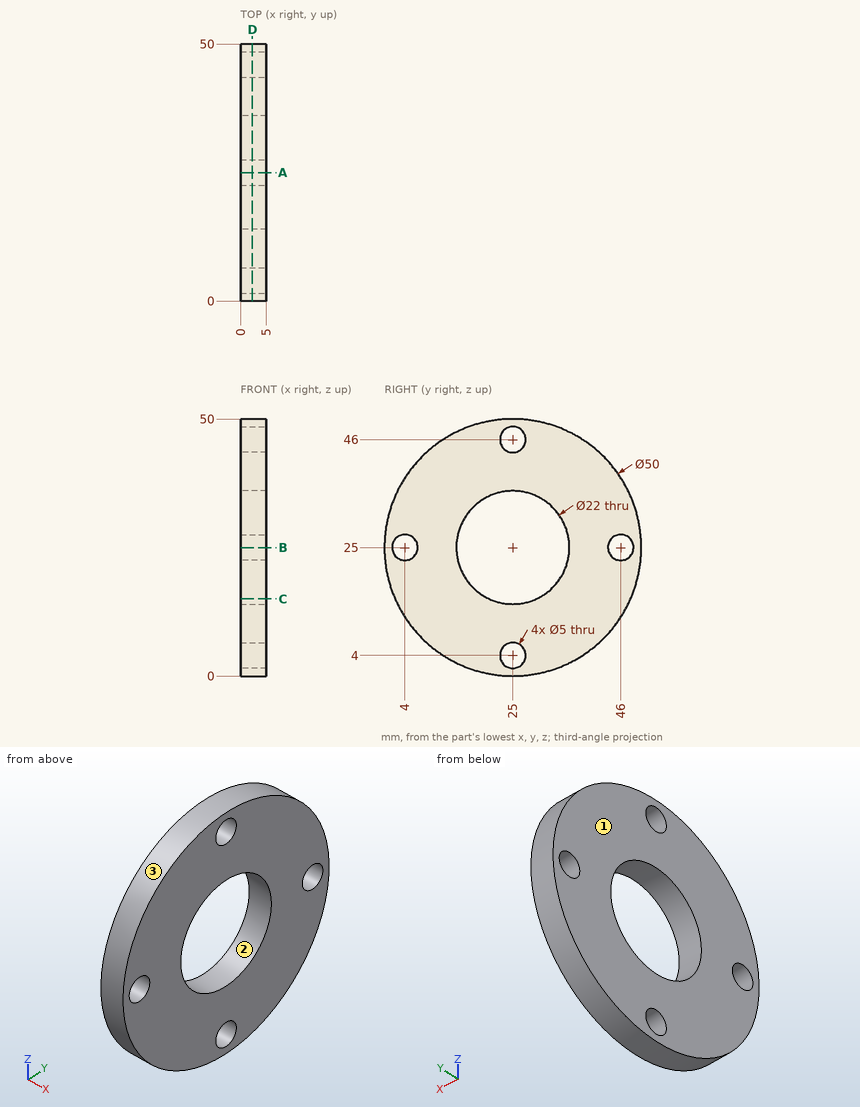
Design review of the part shown in the three views and the two pictorial views. Dimensions are in mm from the part's minimum x, y and z. Round coordinates to 2 decimals unless told otherwise and drop trailing zeros. Write each loop counter-clockwise with the first axis right and the second up, starting at its lowest first coordinate (ties: lowest second). Pieces come first, ordered by that corner, then holes. Notation, with made-up numbers: (65, 87) - (107, 87) arc R23 cw to (107, 110) - close; hole circle Ø9 at (46, 9). An arc over 180 degrees is marked (long way). Return JSON: item names as keys, results as strings. Group by question number.
Item 1: The part is to be moulded in two halves that separate along Y. For the marked faces 1, 2 and 3, say which applies: pulls with the +Y half, pulls with the -Y half, needs draft (parallel to the pull), parting line crosses it, or undercut.
Item 2: Insertion check: P1, Ø2, axis at x = 2.5, y = 34.5, coming from the -Z side; P2, Ø1.5, axis at x = 1.5, y = 29.5, coming from the -Z side. Each pin has a flat end and moves straight along its axis. Give the tip position at first contact, or say it passes through.
Item 3: We need section A-A on y = 25. Write out the cut boundary in (x, z), and give its area (3 significant figures).
Item 4: We need section C-C on z = 15. Write out the cut boundary in (x, y).
Item 5: We need section D-D on x = 2.3. Write out the cut boundary in (y, z).
Item 6: For probe 1 along Y at (x, z) = (1.3, 25); probe 2 along Y at (x, z) = (0.95, 21); probe 3 along Y at (x, z) = (4.15, 24), list the stretches that pass through material, from the lowest coordinate up. Write a range as [from, to].
Model answer:
{
 "1": {"face 1": "needs draft", "face 2": "undercut", "face 3": "parting line crosses it"},
 "2": {"P1": "stops at z = 1.49", "P2": "stops at z = 0.28"},
 "3": {"outline": "(0, 0) - (5, 0) - (5, 1.5) - (0, 1.5) - close; (0, 6.5) - (5, 6.5) - (5, 14) - (0, 14) - close; (0, 36) - (5, 36) - (5, 43.5) - (0, 43.5) - close; (0, 48.5) - (5, 48.5) - (5, 50) - (0, 50) - close", "area": "90.0 mm²"},
 "4": {"outline": "(0, 2.09) - (5, 2.09) - (5, 20.42) - (0, 20.42) - close; (0, 29.58) - (5, 29.58) - (5, 47.91) - (0, 47.91) - close"},
 "5": {"outline": "circle Ø50 at (25, 25); hole circle Ø5 at (4, 25); hole circle Ø22 at (25, 25); hole circle Ø5 at (25, 4); hole circle Ø5 at (25, 46); hole circle Ø5 at (46, 25)"},
 "6": {"probe 1": "y = [0, 1.5], [6.5, 14], [36, 43.5], [48.5, 50]", "probe 2": "y = [0.32, 14.75], [35.25, 49.68]", "probe 3": "y = [0.02, 1.71], [6.29, 14.05], [35.95, 43.71], [48.29, 49.98]"}
}
